Build history of the part. All positions in model axes, mm. A direction names the side the tool comes from. Give positions to 0.01 mm unless a question says otherwise; leave off trailing zeros. Order: outer loops, then holes, each group sorted by start corner. A loop starts at its lowest first (then second) coordinate and runs counter-clockwise, first axis right, second up. Notation, with made-up numbers: (2.5, 38) -> (57.5, 38) arc R13 ccw to (57.5, 51) -> close; hole circle Ø8 at (-21.5, 28). An arc over 180 degrees is marked (long way). Use a Markdown table: item, result. Add a question column.
Solid Edge part; units mm, degrees
sketch "Sketch1" plane through (0, 0, 0) normal (0, 0, 1) x (1, 0, 0)
  line L0 (80, 65) -> (0, 65)
  line L1 (0, 65) -> (0, 0)
  line L2 (0, 0) -> (80, 0)
  line L3 (80, 0) -> (80, 65)
extrude "Protrusion1" add sketch "Sketch1" against normal blind 18
fillet "Redondo_1" radius 3 12 edges at (40, 0, -18) (80, 0, -9) (40, 65, 0) (80, 32.5, 0) (40, 0, 0) (0, 32.5, 0) (80, 32.5, -18) (80, 65, -9) (0, 32.5, -18) (0, 65, -9) (40, 65, -18) (0, 0, -9)
sketch "Sketch2" plane through (40, 32.5, 0) normal (0, 0, 1) x (-1, 0, 0)
  circle A0 centre (30, 15.5) radius 2.5
  circle A1 centre (30, -19.5) radius 2.5
  circle A2 centre (-30, 15.5) radius 2.5
  circle A3 centre (-30, -19.5) radius 2.5
extrude "Recorte_Extrudado_2" cut sketch "Sketch2" against normal blind 7
chamfer "Chanfro_2" distance 0.5 angle 45 4 edges at (12.5, 17, -7) (12.5, 52, -7) (72.5, 52, -7) (72.5, 17, -7)
properties material "PVC"
(1) Band-saw the part on C-C on x = 10. Give the cut face in (y, z).
(2) Band-saw the part on A-A on z = -4.75. Give the cut face in (x, y).
(3) Wall check: probe 1 along X at (y, z) = (17, -4.75); probe 2 along Y at (x, z) = (70, -2.75); probe 3 along Y at (x, z) = (10, -1.25). Give the ranges that are in metal, low to high.
(4) Mould opens along Y. For faces 3 (the face through (0.86, 64.1, -9.08)), 4 (the face through (70.54, 54.44, -3.2)), 5 (the face through (0.86, 32.09, -17.1)), 6 (the face through (10.54, 19.44, -3.2)) say: released by +Y, released by -Y, zero draft, split by the parting line, or undercut.
(5) Tool access for faces 1 (the face through (39, 0, -9)), 2 (the face through (10, 52, -7)): list every direction of +Z, -Z, +X, -X, +Y, -Y with a clear straight run to the whole face (end or side of a thin tool).
(6) Band-saw the part on B-B on y = 17. Give the cut face in (x, z), plus the area to 3 significant figures.
(7) Pin check, flat tips, straight feed: pin 1 Ø4.5 at (x, y) = (70, 17) entering from +Z; pin 2 Ø3 at (x, y) = (70, 52) entering from +Z. Stop position of each tip, or through.
Response:
| question | item | result |
|---|---|---|
| 1 | outline | (0, -15) arc R3 ccw to (3, -18) -> (62, -18) arc R3 ccw to (65, -15) -> (65, -3) arc R3 ccw to (62, 0) -> (54.5, 0) -> (54.5, -6.5) -> (54, -7) -> (50, -7) -> (49.5, -6.5) -> (49.5, 0) -> (19.5, 0) -> (19.5, -6.5) -> (19, -7) -> (15, -7) -> (14.5, -6.5) -> (14.5, 0) -> (3, 0) arc R3 ccw to (0, -3) -> close |
| 2 | outline | (0, 3) arc R3 ccw to (3, 0) -> (77, 0) arc R3 ccw to (80, 3) -> (80, 62) arc R3 ccw to (77, 65) -> (3, 65) arc R3 ccw to (0, 62) -> close; hole circle Ø5 at (10, 17); hole circle Ø5 at (10, 52); hole circle Ø5 at (70, 17); hole circle Ø5 at (70, 52) |
| 3 | probe 1 | x = 0 to 7.5, 12.5 to 67.5, 72.5 to 80 |
| 3 | probe 2 | y = 0.01 to 14.5, 19.5 to 49.5, 54.5 to 64.99 |
| 3 | probe 3 | y = 0.56 to 14.5, 19.5 to 49.5, 54.5 to 64.44 |
| 4 | face 3 | released by +Y |
| 4 | face 4 | undercut |
| 4 | face 5 | zero draft |
| 4 | face 6 | undercut |
| 5 | face 1 | +Z, -Z, +X, -X, -Y |
| 5 | face 2 | +Z |
| 6 | outline | (0, -15) arc R3 ccw to (3, -18) -> (77, -18) arc R3 ccw to (80, -15) -> (80, -3) arc R3 ccw to (77, 0) -> (72.5, 0) -> (72.5, -6.5) -> (72, -7) -> (68, -7) -> (67.5, -6.5) -> (67.5, 0) -> (12.5, 0) -> (12.5, -6.5) -> (12, -7) -> (8, -7) -> (7.5, -6.5) -> (7.5, 0) -> (3, 0) arc R3 ccw to (0, -3) -> close |
| 6 | area | 1,360 mm² |
| 7 | pin 1 | stops at z = -6.75 |
| 7 | pin 2 | stops at z = -7 |
